Autodesk Inventor part; units mm, degrees
ref_plane "YZ Plane" through (0, 0, 0) normal (1, 0, 0) x (0, 1, 0)
ref_plane "XZ Plane" through (0, 0, 0) normal (0, 1, 0) x (-1, 0, 0)
ref_plane "XY Plane" through (0, 0, 0) normal (0, 0, 1) x (1, 0, 0)
sketch "Boceto1" plane through (0, 0, 0) normal (0, 1, 0) x (-1, 0, 0)
  line L0 (0, 0) -> (50, 0)
  line L1 (50, 0) -> (50, -65)
  line L2 (50, -65) -> (0, -65)
  line L3 (0, -65) -> (0, 0)
  line L4 (17.7, -45) -> (32.7, -45)
  line L5 (32.7, -45) -> (32.7, -20)
  line L6 (32.7, -20) -> (17.7, -20)
  line L7 (17.7, -20) -> (17.7, -45)
  line L8 (17.7, -45) -> (32.7, -20) construction
  line L9 (32.7, -45) -> (17.7, -20) construction
  line L10 (35.7, -17) -> (35.7, -48)
  line L11 (35.7, -48) -> (14.7, -48)
  line L12 (14.7, -48) -> (14.7, -17)
  line L13 (14.7, -17) -> (35.7, -17)
  line L14 (41, -1.5) -> (9, -1.5)
  line L15 (9, -1.5) -> (9, -14)
  line L16 (9, -14) -> (41, -14)
  line L17 (41, -14) -> (41, -1.5)
  line L18 (32.7, -32.5) -> (17.7, -32.5) construction
  line L19 (41, -7.75) -> (35.5, -7.75) construction
  line L20 (35.5, -7.75) -> (14.5, -7.75) construction
  line L21 (14.5, -7.75) -> (9, -7.75) construction
  circle A0 centre (35.5, -7.75) radius 1.4
  circle A1 centre (14.5, -7.75) radius 1.4
  line L22 (41, -63.5) -> (9, -63.5)
  line L23 (9, -63.5) -> (9, -51)
  line L24 (9, -51) -> (41, -51)
  line L25 (41, -51) -> (41, -63.5)
  circle A2 centre (35.5, -57.25) radius 1.4
  circle A3 centre (14.5, -57.25) radius 1.4
  line L26 (50, -32.5) -> (43.2, -32.5) construction
  line L27 (0, -32.5) -> (6.8, -32.5)
  line L28 (45.9347, 0) -> (45.9347, -15.5) construction
  line L29 (43.2, -32.5) -> (43.2, -14.5) construction
  line L30 (43.2, -14.5) -> (50, -14.5) construction
  circle A4 centre (43.2, -14.5) radius 1.4
  line L31 (25.2, -20) -> (25.2, -45) construction
  circle A5 centre (7.2, -14.5) radius 1.4
  circle A6 centre (35.5, -57.25) radius 1.4
  circle A7 centre (43.2, -50.5) radius 1.4
  circle A8 centre (7.2, -50.5) radius 1.4
  point P0 (25.2, -32.5)
  point P1 (25, -14)
  point P2 (25.2, -17)
  dimension "d0" = 65
  dimension "d1" = 50
  dimension "d2" = 25
  dimension "d3" = 15
  dimension "d4" = 3
  dimension "d5" = 12.5
  dimension "d6" = 32
  dimension "d7" = 3
  dimension "d8" = 5.5
  dimension "d9" = 5.5
  dimension "d10" = 2.8
  dimension "d11" = 2.8
  dimension "d12" = 6.8
  dimension "d13" = 6.8
  dimension "d15" = 2.8
  dimension "d30" = 1.5
  dimension "d31" = 36
  dimension "d32" = 36
extrude "Extrusión1" add sketch "Boceto1" along normal blind 3 contours L10 L11 L12 L13
extrude "Extrusión2" add sketch "Boceto1" against normal blind 4 contours L0 L1 L2 L3 | L17 L16 L15 L14 | L22 L23 L24 L25
extrude "Extrusión3" add sketch "Boceto1" along normal blind 1.5 contours L17 L16 L15 L14 | L22 L23 L24 L25
sketch "Boceto2" plane through (0, 1.5, 0) normal (0, 1, 0) x (1, 0, 0)
  line L0 (-41, 1.5) -> (-9, 1.5)
  line L1 (-25, 1.5) -> (-25, 14)
  line L2 (-9, 14) -> (-41, 14)
  line L3 (-20, 1.5) -> (-30, 1.5)
  line L4 (-30, 1.5) -> (-30, 14)
  line L5 (-30, 14) -> (-20, 14)
  line L6 (-20, 14) -> (-20, 1.5)
  line L7 (-20, 1.5) -> (-30, 14) construction
  line L8 (-30, 1.5) -> (-20, 14) construction
  line L9 (-32.7, 32.5) -> (-17.7, 32.5) construction
  line L10 (-41, 63.5) -> (-9, 63.5)
  line L11 (-9, 51) -> (-41, 51)
  line L12 (-30, 63.5) -> (-30, 51)
  line L13 (-20, 51) -> (-20, 63.5)
  point P0 (0, 0)
  point P1 (-25, 7.75)
  dimension "d22" = 10
extrude "Extrusión4" cut sketch "Boceto2" against normal blind 0.75
extrude "Extrusión5" add sketch "Boceto1" against normal blind 4 contours L7 L6 L5 L4 | L10 L11 L12 L13
sketch "Boceto3" plane through (0, 3, 0) normal (0, 1, 0) x (1, 0, 0)
  line L0 (-25.2, 20) -> (-25.2, 45) construction
  line L1 (-35.7, 17) -> (-14.7, 17)
  line L2 (-25.2, 17) -> (-25.2, 48)
  line L3 (-14.7, 48) -> (-35.7, 48)
  line L4 (-24.95, 17) -> (-25.45, 17)
  line L5 (-25.45, 17) -> (-25.45, 48)
  line L6 (-25.45, 48) -> (-24.95, 48)
  line L7 (-24.95, 48) -> (-24.95, 17)
  line L8 (-24.95, 17) -> (-25.45, 48) construction
  line L9 (-25.45, 17) -> (-24.95, 48) construction
  point P0 (0, 0)
  point P1 (-25.2, 32.5)
  point P2 (-24.95, 48)
  point P3 (-25.45, 17)
  dimension "d27" = 0.5
extrude "Extrusión6" cut sketch "Boceto3" against normal blind 1.5
fillet "Empalme1" radius 2 4 edges at (-41, 0.75, -51) (-9, 0.75, -51) (-9, 0.75, -14) (-41, 0.75, -14)
equation "\"d9\" = d8"
equation "\"d13\" = d12"
properties part number "Molde 1FBR 1.5mm"
The model under review builds one solid part; all positions refer to its coordinate system, in mm. A direction names the side the tool comes from. Give positions to 0.01 mm unless a question says otherwise; leave off trailing zeros. Order: outer loops, then holes, each group sorted by start corner. A loop starts at its lowest first (then second) coordinate and runs counter-clockwise, first axis right, second up. Notation, with made-up numbers: M 6,-39 L 35,-39 A14 ccw 35,-24 Z; hole C 45.5,54 d7. An arc over 180 degrees is marked long. Answer in a Markdown table with one row per item. Add a question column.
1. Add section D-D on x = -17. State the section outline as (y, z) points, plus the area to 4 significant figures.
2. Machinability: for faces 4 (the flat face through (-25, 0.75, -57)), 5 (the flat face through (-24.8, 0.6, -51)), 6 (the flat face through (-25, 1, -45)), 7 (the flat face through (-14, 1.5, -6)), which of the approach directions +Z, -Z, +X, -X, +Y, -Y give a long, thin tool a straight path to every point of the face, cutting with its end or side? Answer none if there is none.
3. For pin 1 Ø0.9 at (x, y) = (-25.5, 1.5) entering from -Z; pin 2 Ø8 at (x, z) = (-6, -26) entering from +Y; pin 3 Ø3.5 at (x, z) = (-36, -59) entering from +Y, all flat-tipped, find the tip position at first contact; note any pin that passes through.
4. Add section B-B on z = -7.75. State the section outline as (x, y) points.
5. Mouldability with a two-part tool opening along X and no side actions: class faces 1 (the cylindrical face through (-9.6, 0.76, -51.57)), 2 (the cylindrical face through (-7.95, -1.97, -13.32)), 3 (the flat face through (-36, 0, -32)) as released by +X, released by -X, zero draft, split by the parting line, or undercut.
6. Add section C-C on y = -1. Count the separate pieces of the cut face and the enclosed holes in it, plus the area to 3 significant figures.
7. To check wall thickness, follow line 1 along Z through (x, y) = (-7.2, -1.2); line 2 along Z through (x, y) = (-32, 1.25); line 3 along X through (y, z) = (-3, -49.5). State the ranges of each line that lie inside material, in increasing order.
8. Add section A-A on x = -43.2. State the section outline as (y, z) points, plus the area to 3 significant figures.
The answers:
| question | item | result |
|---|---|---|
| 1 | outline | M -4,-65 L 0,-65 L 0,-63.5 L 1.5,-63.5 L 1.5,-51 L 0,-51 L 0,-48 L 3,-48 L 3,-17 L 0,-17 L 0,-14 L 1.5,-14 L 1.5,-1.5 L 0,-1.5 L 0,0 L -4,0 Z |
| 1 | area | 390.5 mm2 |
| 2 | face 4 | -Z, +Y |
| 2 | face 5 | +X, -X, +Y |
| 2 | face 6 | +Y |
| 2 | face 7 | +Z, +X, -X, +Y |
| 3 | pin 1 | z = -48 |
| 3 | pin 2 | y = 0 |
| 3 | pin 3 | y = 1.5 |
| 4 | outline | M -50,-4 L -36.9,-4 L -36.9,1.5 L -41,1.5 L -41,0 L -50,0 Z; M -34.1,-4 L -15.9,-4 L -15.9,1.5 L -20,1.5 L -20,0.75 L -30,0.75 L -30,1.5 L -34.1,1.5 Z; M -13.1,-4 L 0,-4 L 0,0 L -9,0 L -9,1.5 L -13.1,1.5 Z |
| 5 | face 1 | released by +X |
| 5 | face 2 | undercut |
| 5 | face 3 | zero draft |
| 6 | separate pieces | 1 |
| 6 | enclosed holes | 8 |
| 6 | area | 3,200 mm2 |
| 7 | line 1 | -65 to -51.9, -49.1 to -15.9, -13.1 to 0 |
| 7 | line 2 | -63.5 to -51, -48 to -45, -20 to -17, -14 to -1.5 |
| 7 | line 3 | -50 to -44.18, -42.22 to -8.18, -6.22 to 0 |
| 8 | outline | M -4,-65 L 0,-65 L 0,-51.9 L -4,-51.9 Z; M -4,-49.1 L 0,-49.1 L 0,-15.9 L -4,-15.9 Z; M -4,-13.1 L 0,-13.1 L 0,0 L -4,0 Z |
| 8 | area | 238 mm2 |
